from build123d import *

# Parameters (mm, degrees)
SKETCH3_R           = 3.175
BOSS_EXTRUDE1_DEPTH = 3.302
CUT_SWEEP1_PITCH    = 1.27
SKETCH8_R           = 2.2225
BOSS_EXTRUDE3_DEPTH = 9.398
SKETCH10_R          = 1.905
BOSS_EXTRUDE5_DEPTH = 3.429
SKETCH11_R          = 4.445
BOSS_EXTRUDE6_DEPTH = 0.127
DOME1_FACE_RADIUS   = 4.445
DOME1_HEIGHT        = 2.54


with BuildPart() as part:
    # Sketch3 → Boss-Extrude1 (new body)
    with BuildSketch(Plane.XY):
        with Locations(Location((0, 0, 0), (0, 0, 180))):
            Circle(SKETCH3_R)
    extrude(amount=BOSS_EXTRUDE1_DEPTH)

    # Cut-Sweep1: arcs per turn and ends read off the stored shape
    # Cut-Sweep1: the profile of Sketch5 profile screwed along a left-hand helix through 4.5 turns, 8 arcs to a turn; built about Z, then put on its axis
    cut_sweep1_z = Axis((0, 0, 0), (0, 0, 1))
    cut_sweep1_corners = [(2.54, 0, -1.397), (3.1753, 0, -1.763790626), (3.1753, 0, -0.776209374), (2.54, 0, -1.143)]
    with BuildLine(mode=Mode.PRIVATE) as cut_sweep1_profile:
        Line(cut_sweep1_corners[0], cut_sweep1_corners[1])
        Line(cut_sweep1_corners[1], cut_sweep1_corners[2])
        Line(cut_sweep1_corners[2], cut_sweep1_corners[3])
        Line(cut_sweep1_corners[3], cut_sweep1_corners[0])
    cut_sweep1_cap = Face(cut_sweep1_profile.wire())
    cut_sweep1_turn_angles = [0, -22.5, -45, -67.5, -90, -112.5, -135, -157.5, -180, -202.5, -225, -247.5, -270, -292.5, -315, -337.5, -360]
    cut_sweep1_turn_weights = [1, 0.9238795325112867, 1, 0.9238795325112867, 1, 0.9238795325112867, 1, 0.9238795325112867, 1, 0.9238795325112867, 1, 0.9238795325112867, 1, 0.9238795325112867, 1, 0.9238795325112867, 1]
    cut_sweep1_turn_rails = [Edge.make_bspline([Vector(p[0], p[1], 0).rotate(cut_sweep1_z, cut_sweep1_turn_angles[k]) / cut_sweep1_turn_weights[k] + Vector(0, 0, p[2] + -CUT_SWEEP1_PITCH * cut_sweep1_turn_angles[k] / 360) for k in range(17)], [0, 0, 0, 1, 1, 2, 2, 3, 3, 4, 4, 5, 5, 6, 6, 7, 7, 8, 8, 8], 2, cut_sweep1_turn_weights) for p in cut_sweep1_corners]
    cut_sweep1_turn_sides = [Face.make_surface_from_curves(cut_sweep1_turn_rails[p[0]], cut_sweep1_turn_rails[p[1]]) for p in [(0, 1), (1, 2), (2, 3), (3, 0)]]
    cut_sweep1_last_angles = [-1440, -1462.5, -1485, -1507.5, -1530, -1552.5, -1575, -1597.5, -1620]
    cut_sweep1_last_weights = [1, 0.9238795325112867, 1, 0.9238795325112867, 1, 0.9238795325112867, 1, 0.9238795325112867, 1]
    cut_sweep1_last_rails = [Edge.make_bspline([Vector(p[0], p[1], 0).rotate(cut_sweep1_z, cut_sweep1_last_angles[k]) / cut_sweep1_last_weights[k] + Vector(0, 0, p[2] + -CUT_SWEEP1_PITCH * cut_sweep1_last_angles[k] / 360) for k in range(9)], [0, 0, 0, 1, 1, 2, 2, 3, 3, 4, 4, 4], 2, cut_sweep1_last_weights) for p in cut_sweep1_corners]
    cut_sweep1_last_sides = [Face.make_surface_from_curves(cut_sweep1_last_rails[p[0]], cut_sweep1_last_rails[p[1]]) for p in [(0, 1), (1, 2), (2, 3), (3, 0)]]
    cut_sweep1 = Plane(origin=(0, 0, 0), x_dir=(0, 1, 0), z_dir=(0, 0, 1)) * Solid(Shell([*[p.moved(Location((0, 0, CUT_SWEEP1_PITCH * i))) for i in range(4) for p in cut_sweep1_turn_sides], *cut_sweep1_last_sides, cut_sweep1_cap, cut_sweep1_cap.rotate(cut_sweep1_z, -1620).moved(Location((0, 0, -CUT_SWEEP1_PITCH * -1620 / 360)))]))
    add(cut_sweep1, mode=Mode.SUBTRACT)

    # Sketch8 → Boss-Extrude3 (add)
    with BuildSketch(Plane.XY):
        Circle(SKETCH8_R)
    extrude(amount=-BOSS_EXTRUDE3_DEPTH)

    # Sketch10 → Boss-Extrude5 (add)
    with BuildSketch(Plane(origin=(0, 0, -9.398), x_dir=(-1, 0, 0), z_dir=(0, 0, -1))):
        with Locations(Location((0, 0, 0), (0, 0, 180))):
            Circle(SKETCH10_R)
    extrude(amount=BOSS_EXTRUDE5_DEPTH)

    # Sketch11 → Boss-Extrude6 (add)
    with BuildSketch(Plane.XY.offset(3.302)):
        Circle(SKETCH11_R)
    extrude(amount=BOSS_EXTRUDE6_DEPTH)

    # Dome1: a dome of height H over a round flat face of radius A is a cap of a sphere of radius (A * A + H * H) / (2 * H)
    dome1_r = (DOME1_FACE_RADIUS * DOME1_FACE_RADIUS + DOME1_HEIGHT * DOME1_HEIGHT) / (2 * DOME1_HEIGHT)
    dome1_base = Plane((0, 0, 3.429), z_dir=(0, 0, 1))
    with Locations(dome1_base.offset(DOME1_HEIGHT - dome1_r)):
        dome1_ball = Sphere(dome1_r, mode=Mode.PRIVATE)
    add(split(dome1_ball, bisect_by=dome1_base, keep=Keep.TOP, mode=Mode.PRIVATE))


solid = part.part
Build history of the part. All positions in model axes, mm. A direction names the side the tool comes from. Coordinates: 2 decimals unless noted, no trailing zeros. Write each loop counter-clockwise with the first axis right and the second up, starting at its lowest first coordinate (ties: lowest second). Pieces come first, ordered by that corner, then holes.
(1) Pin check, flat tips, straight feed: pin 1 Ø1 at (x, y) = (1.5, -1.5) entering from +Z; pin 2 Ø5 at (y, z) = (1.5, -8.5) entering from -X; pin 3 Ø5 at (x, z) = (2, -3) entering from -Y. Stop position of each tip, or through.
(2) 3-axis set-ups, long thin cutter, end or side, ignore diameter. For faces 1 (the flat face through (-2, -2, 3.302)), 2 (the flat face through (-0.2, -2.4, 0)), 3 (the flat face through (0, 0, -12.827)): which of +Z, -Z, +X, -X, +Y, -Y reach the whole face in a straight line?
(3) Cut at C-C on x = 3.75. List the corners of the cut face in (y, z).
(4) Drill centre lines: line 1 (Z direction, x = -3, y = 0); line 2 (Z direction, x = 3, y = 0); line 3 (Y direction, x = 2.25, z = 5). Where is each one in solid material? Low to high.
(5) Cut at B-B on y = -4. List the corners of the cut face in (x, z), and give its area (3 significant figures).
(6) Cut at A-A on z = -2. List the corners of the cut face in (x, y) (1 decimal), and give its area (3 significant figures).
(7) Cut at D-D on z = -11. List the corners of the cut face in (x, y) (3 decimals), and give its area (3 significant figures).
Working result:
1. pin 1: stops at z = 5.71
1. pin 2: stops at x = -2.22
1. pin 3: stops at y = -2.22
2. face 1: none
2. face 2: -Z
2. face 3: -Z, +X, -X, +Y, -Y
3. outline: (-2.39, 3.3) - (2.39, 3.3) - (2.39, 3.43) arc R3.54 ccw to (-2.39, 3.43) - close
4. line 1: z = 0.08 to 0.56, 1.35 to 1.83, 2.62 to 3.1, 3.3 to 5.01
4. line 2: z = 0.71 to 1.19, 1.98 to 2.46, 3.25 to 5.01
4. line 3: y = -2 to 2
5. outline: (-1.94, 3.3) - (1.94, 3.3) - (1.94, 3.43) arc R3.26 ccw to (-1.94, 3.43) - close
5. area: 2.18 mm2
6. outline: circle Ø4.4 at (0, 0)
6. area: 15.5 mm2
7. outline: circle Ø3.81 at (0, 0)
7. area: 11.4 mm2
